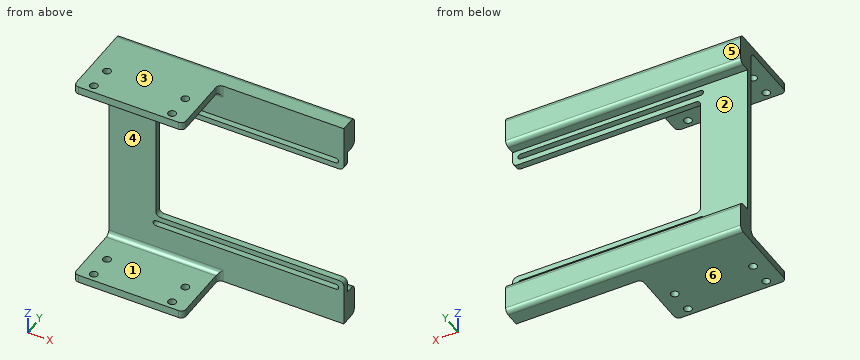
```python
from build123d import *

# Parameters (mm, degrees)
SKETCH1_W               = 150
SKETCH1_H               = 140
BOSS_EXTRUDE1_DEPTH     = 12
SKETCH4_W               = 70
SKETCH4_H               = 140
BOSS_EXTRUDE2_DEPTH     = 40
SKETCH5_R               = 2.5
CUT_EXTRUDE1_DEPTH      = 141
SKETCH7_W               = 150
SKETCH7_H               = 100
CUT_EXTRUDE2_DEPTH      = 8
SKETCH8_W               = 120
SKETCH8_H               = 80
CUT_EXTRUDE3_DEPTH      = 41
CUT_EXTRUDE3_DEPTH_BACK = 13
CUT_EXTRUDE4_DEPTH      = 45
SKETCH11_W              = 130
SKETCH11_H              = 40
CUT_EXTRUDE6_DEPTH      = 71
FILLET5_R               = 3
FILLET6_R               = 3
FILLET7_R               = 3
FILLET8_R               = 3
FILLET9_R               = 3
FILLET10_R              = 3
FILLET11_R              = 3


with BuildPart() as part:
    # Sketch1 → Boss-Extrude1 (new body)
    with BuildSketch(Plane(origin=(0, 0, 0), x_dir=(1, 0, 0), z_dir=(0, 1, 0))):
        Rectangle(SKETCH1_W, SKETCH1_H)
    extrude(amount=BOSS_EXTRUDE1_DEPTH)

    # Sketch4 → Boss-Extrude2 (add)
    with BuildSketch(Plane.XZ):
        with Locations((-40, 0)):
            Rectangle(SKETCH4_W, SKETCH4_H)
    extrude(amount=BOSS_EXTRUDE2_DEPTH)

    # Sketch5 → Cut-Extrude1 (cut, through all)
    with BuildSketch(Plane.XY.offset(70)):
        with Locations((-65, -35)):
            Circle(SKETCH5_R)
        with Locations((-15, -35)):
            Circle(SKETCH5_R)
        with Locations((-15, -20)):
            Circle(SKETCH5_R)
        with Locations((-65, -20)):
            Circle(SKETCH5_R)
    extrude(amount=-CUT_EXTRUDE1_DEPTH, mode=Mode.SUBTRACT)

    # Sketch7 → Cut-Extrude2 (cut)
    with BuildSketch(Plane(origin=(0, 12, 0), x_dir=(1, 0, 0), z_dir=(0, 1, 0))):
        Rectangle(SKETCH7_W, SKETCH7_H)
    extrude(amount=-CUT_EXTRUDE2_DEPTH, mode=Mode.SUBTRACT)

    # Sketch8 → Cut-Extrude3 (cut, two sides)
    with BuildSketch(Plane.XZ) as cut_extrude3_sk:
        with Locations((15, 0)):
            Rectangle(SKETCH8_W, SKETCH8_H)
    extrude(amount=CUT_EXTRUDE3_DEPTH, mode=Mode.SUBTRACT)
    extrude(cut_extrude3_sk.sketch, amount=-CUT_EXTRUDE3_DEPTH_BACK, mode=Mode.SUBTRACT)

    # Sketch9 → Cut-Extrude4 (cut, through all)
    with BuildSketch(Plane(origin=(0, 4, 0), x_dir=(1, 0, 0), z_dir=(0, 1, 0))):
        with BuildLine():
            Line((-45, 47), (70, 47))
            ThreePointArc((70, 47), (71.75, 45.25), (70, 43.5))
            Line((70, 43.5), (-45, 43.5))
            ThreePointArc((-45, 43.5), (-46.75, 45.25), (-45, 47))
        make_face()
        with BuildLine():
            Line((-45, -47), (70, -47))
            ThreePointArc((70, -47), (71.75, -45.25), (70, -43.5))
            Line((70, -43.5), (-45, -43.5))
            ThreePointArc((-45, -43.5), (-46.75, -45.25), (-45, -47))
        make_face()
    extrude(amount=-CUT_EXTRUDE4_DEPTH, mode=Mode.SUBTRACT)

    # Sketch11 → Cut-Extrude6 (cut, through all)
    with BuildSketch(Plane(origin=(-5, 0, 0), x_dir=(0, 0, -1), z_dir=(1, 0, 0))):
        with Locations((0, -20)):
            Rectangle(SKETCH11_W, SKETCH11_H)
    extrude(amount=-CUT_EXTRUDE6_DEPTH, mode=Mode.SUBTRACT)

    # Fillet5
    fillet5_edges = [part.edges().sort_by_distance(p)[0] for p in [
        (-40, 0, -65),
        (-40, 0, 65),
    ]]
    fillet(fillet5_edges, radius=FILLET5_R)

    # Fillet6
    fillet6_edges = [part.edges().sort_by_distance(p)[0] for p in [
        (-5, 0, -67.5),
        (-5, 0, 67.5),
    ]]
    fillet(fillet6_edges, radius=FILLET6_R)

    # Fillet7
    fillet7_edges = [part.edges().sort_by_distance(p)[0] for p in [
        (0, 12, 70),
        (0, 12, -70),
    ]]
    fillet(fillet7_edges, radius=FILLET7_R)

    # Fillet8
    fillet8_edges = [part.edges().sort_by_distance(p)[0] for p in [
        (0, 12, -50),
        (0, 12, 50),
    ]]
    fillet(fillet8_edges, radius=FILLET8_R)

    # Fillet9
    fillet9_edges = [part.edges().sort_by_distance(p)[0] for p in [
        (-5, -40, 67.5),
        (-75, -40, -67.5),
        (-75, -40, 67.5),
        (-5, -40, -67.5),
    ]]
    fillet(fillet9_edges, radius=FILLET9_R)

    # Fillet10
    fillet10_edges = [part.edges().sort_by_distance(p)[0] for p in [
        (-45, 2, 40),
        (-45, 2, -40),
    ]]
    fillet(fillet10_edges, radius=FILLET10_R)

    # Fillet11
    fillet11_edges = [part.edges().sort_by_distance(p)[0] for p in [
        (75, 2, 40),
        (75, 2, -40),
    ]]
    fillet(fillet11_edges, radius=FILLET11_R)


solid = part.part
```
Could you check a few things on this model? Use its own coordinates, in mm. Face numbers are marked on the shaded views. A direction names the side the tool comes from. Round coordinates to 2 decimals unless told otherwise and drop trailing zeros. Order: outer loops, then holes, each group sorted by start corner. A loop starts at its lowest first (then second) coordinate and runs counter-clockwise, first axis right, second up. Notation, with made-up numbers: M 7,9.25 L 19,9.25 A33 ccw 19,41.25 Z; hole C -29.5,80 d1. An arc over 180 degrees is marked long. One line per question, with ' | ' between items. Start each with the question number.
(1) Suppose I cut it at D-D on y = -35. List the corners of the cut face in (x, z) for me, then the cut area to 3 significant figures.
(2) Suppose I cut it at C-C on z = -45.25. List the corners of the cut face in (x, y) for me, then the cut area to 3 significant figures.
(3) For the marked faces 1, 2 and 3, which set-ups out of +Z, -Z, +X, -X, +Y, -Y let a thin tool reach every point of the face, with its end or its side?
(4) For P1, Ø1.2, axis at y = 3, z = -18.5, coming from the +X side; P2, Ø5.5, axis at y = -13, z = 68.5, coming from the +X side; P3, Ø2, axis at x = -55, z = -9, coming from the -Y side, each with a flat end and sliding along its axis, tell me the tip position at first contact or that it passes through.
(5) Thinking about a two-plate mould opening in Z: for the marked faces 4, 5 and 6, which applies, +Z half, -Z half, draft (parallel to the pull), parting line (faces both ways), or undercut?
(6) Suppose I cut it at A-A on x = -30. Count the separate pieces of the cut face and the enclosed holes in it, then the cut area to 3 significant figures.
(7) Please list where these lines run through material, in increasing order: line 1 along Z through (x, y) = (-52, -8); line 2 along Z through (x, y) = (20, 5); line 3 along Y through (x, z) = (-15, 66.55).
Geometry results:
1) outline: M -75,-70 L -67.5,-70 L -67.5,-65 L -75,-65 Z; M -75,65 L -67.5,65 L -67.5,70 L -75,70 Z; M -62.5,-70 L -17.5,-70 L -17.5,-65 L -62.5,-65 Z; M -62.5,65 L -17.5,65 L -17.5,70 L -62.5,70 Z; M -12.5,-70 L -5,-70 L -5,-65 L -12.5,-65 Z; M -12.5,65 L -5,65 L -5,70 L -12.5,70 Z | area: 600 mm²
2) outline: M -75,0 L -46.75,0 L -46.75,4 L -75,4 Z; M 71.75,0 L 75,0 L 75,4 L 71.75,4 Z | area: 126 mm²
3) face 1: +X, -X, -Y | face 2: +X, -X, +Y | face 3: +Z, +X, -X, +Y, -Y
4) P1: x = -45 | P2: x = -5 | P3: y = 0
5) face 4: undercut | face 5: draft | face 6: -Z half
6) separate pieces: 4 | enclosed holes: 0 | area: 928 mm²
7) line 1: -70 to -65, 65 to 70 | line 2: -70 to -50, 50 to 70 | line 3: -40 to -37.5, -32.5 to -22.5, -17.5 to 12
